Verification items for the finished model (mm, model axes). A direction names the side the tool comes from. Coordinates: 2 decimals unless noted, no trailing zeros. Order: outer loops, then holes, each group sorted by start corner. A loop starts at its lowest first (then second) coordinate and runs counter-clockwise, first axis right, second up. Notation, with made-up numbers: M 24.5,35 L 76.5,35 A28 ccw 76.5,57 Z; hole C 37,84.25 d3. An arc over 180 degrees is marked long. Answer as a JSON object with one key per item and string values. Group by question number.
(1) Cross-section at C-C (x = -6). Enter the section's corners in (y, z), plus the area to 3 significant figures.
(2) Gauge pin test, flat ends, axial feed: pin 1 Ø1.7 at (y, z) = (4.5, 2.5) entering from -X; pin 2 Ø1.2 at (y, z) = (4.5, 2) entering from +X; pin 3 Ø1.8 at (x, y) = (-5.92, -5.92) entering from -Z; pin 4 Ø2 at (y, z) = (15, 2.5) entering from -X. Record the tip position at first contact, or that the pin passes through.
(3) Access from +Z, -Z, +X, -X, +Y, -Y to the whole of each face (thin tool, end or side, straight path). Record for faces 1 (the face through (0, 5.237, 2)), 2 (the face through (3.15, 14, 2)), 3 (the face through (-2.36, -14.53, 2.46)), 4 (the face through (0, 16.355, 2)).
(4) Cross-section at A-A (x = 0). Enter the section's corners in (y, z), plus the area to 3 significant figures.
(5) Material ranges on line 1 (Y direction, x = 0, z = 2.5); line 2 (Y direction, x = -5, z = 2.5); line 3 (X direction, y = 0, z = 0.5), recorded low to high.
(6) Cross-section at D-D (z = 2). Enter the section's corners in (x, y), plus the area to 3 significant figures.
(7) Cross-section at B-B (y = 0). Enter the section's corners in (x, z).
(8) Mould release check, pull along Y, two halves, no side actions. Record for faces 5 (the face through (6.08, -15.15, 2.46)), 6 (the face through (7.308, -6.497, 1.549)), 7 (the face through (-4.3, -0.3, -2)): released by +Y, released by -Y, zero draft, split by the parting line, or undercut.
from build123d import *

# Parameters (mm, degrees)
F1_DEPTH = 5
F2_R     = 18
F3_DEPTH = 2
F4_R     = 1.5
F5_DEPTH = 7


with BuildPart() as f1:
    # F0 (on Top) → F1 (new body)
    with BuildSketch(Plane.XY):
        with BuildLine():
            Line((9.15, -13.908354), (7.649261, -10.200554))
            ThreePointArc((7.649261, -10.200554), (12.50366, 2.49419), (3.15, 12.354756))
            Line((3.15, 12.354756), (3.15, 16.354756))
            Line((3.15, 16.354756), (0, 16.354756))
            Line((0, 16.354756), (-3.15, 16.354756))
            Line((-3.15, 16.354756), (-3.15, 12.354756))
            ThreePointArc((-3.15, 12.354756), (-12.50366, 2.49419), (-7.649261, -10.200554))
            Line((-7.649261, -10.200554), (-9.15, -13.908354))
            Line((-9.15, -13.908354), (-3.1, -16.357103))
            Line((-3.1, -16.357103), (-1.599261, -12.649303))
            ThreePointArc((-1.599261, -12.649303), (0, -12.75), (1.599261, -12.649303))
            Line((1.599261, -12.649303), (3.1, -16.357103))
            Line((3.1, -16.357103), (9.15, -13.908354))
        make_face()
    extrude(amount=F1_DEPTH)

    # F2 (on face) → F3 (join)
    with BuildSketch(Plane(origin=(0, 0, 0), x_dir=(1, 0, 0), z_dir=(0, 0, -1))):
        Circle(F2_R)
    extrude(amount=F3_DEPTH)

    # F4 (on face) → F5 (cut, through all)
    with BuildSketch(Plane.XY.offset(5)):
        with BuildLine():
            Line((-1.55, 5.237479), (-1.55, 3.687479))
            ThreePointArc((-1.55, 3.687479), (0, -4), (1.55, 3.687479))
            Line((1.55, 3.687479), (1.55, 5.237479))
            Line((1.55, 5.237479), (0, 5.237479))
            Line((0, 5.237479), (-1.55, 5.237479))
        make_face()
        with Locations((-5.922019, 5.922019)):
            Circle(F4_R)
        with Locations((-5.922019, -5.922019)):
            Circle(F4_R)
        with Locations((5.922019, -5.922019)):
            Circle(F4_R)
        with Locations((5.922019, 5.922019)):
            Circle(F4_R)
    extrude(amount=-F5_DEPTH, mode=Mode.SUBTRACT)


solid = f1.part
Taken from the geometry:
{
 "1": {"outline": "M -16.97,-2 L -7.42,-2 L -7.42,5 L -15.18,5 L -15.18,0 L -16.97,0 Z; M -4.42,-2 L 4.42,-2 L 4.42,5 L -4.42,5 Z; M 7.42,-2 L 16.97,-2 L 16.97,0 L 11.25,0 L 11.25,5 L 7.42,5 Z", "area": "158 mm²"},
 "2": {"pin 1": "stops at x = -12.22", "pin 2": "stops at x = 12.14", "pin 3": "passes through", "pin 4": "stops at x = -3.15"},
 "3": {"face 1": "+Z, -Z", "face 2": "+Z, +X, +Y", "face 3": "+Z, -Y", "face 4": "+Z, +X, -X, +Y"},
 "4": {"outline": "M -18,-2 L -4,-2 L -4,5 L -12.75,5 L -12.75,0 L -18,0 Z; M 5.24,-2 L 18,-2 L 18,0 L 16.35,0 L 16.35,5 L 5.24,5 Z", "area": "153 mm²"},
 "5": {"line 1": "y = -12.75 to -4, 5.24 to 16.35", "line 2": "y = -15.59 to -7.11, -4.74 to 4.74, 7.11 to 11.73", "line 3": "x = -12.75 to -4, 4 to 12.75"},
 "6": {"outline": "M -9.15,-13.91 L -3.1,-16.36 L -1.6,-12.65 A12.75 ccw 1.6,-12.65 L 3.1,-16.36 L 9.15,-13.91 L 7.65,-10.2 A12.75 ccw 3.15,12.35 L 3.15,16.35 L -3.15,16.35 L -3.15,12.35 A12.75 ccw -7.65,-10.2 Z; hole C -5.92,-5.92 d3; hole C -5.92,5.92 d3; hole M -1.55,3.69 A4 ccw long 1.55,3.69 L 1.55,5.24 L -1.55,5.24 Z; hole C 5.92,-5.92 d3; hole C 5.92,5.92 d3", "area": "500 mm²"},
 "7": {"outline": "M -18,-2 L -4,-2 L -4,5 L -12.75,5 L -12.75,0 L -18,0 Z; M 4,-2 L 18,-2 L 18,0 L 12.75,0 L 12.75,5 L 4,5 Z"},
 "8": {"face 5": "released by -Y", "face 6": "undercut", "face 7": "zero draft"}
}
